from build123d import *

# Parameters (mm, degrees)
SKETCH_1_R      = 1
SKETCH_1_R_2    = 0.75
EXTRUDE_1_DEPTH = 0.5
SKETCH_1_4_R    = 0.75
SKETCH_1_4_R_2  = 0.45
EXTRUDE_2_DEPTH = 9
SKETCH_1_6_R    = 0.45
EXTRUDE_3_DEPTH = 10
CHAMFER_3_SIZE  = 0.1
CHAMFER_4_SIZE  = 0.1
CHAMFER_5_SIZE  = 0.1


with BuildPart() as part:
    # 草图1 → 凸台-拉伸1 (new body)
    with BuildSketch(Plane(origin=(0, 0, 0), x_dir=(1, 0, 0), z_dir=(0, 1, 0))):
        Circle(SKETCH_1_R)
        Circle(SKETCH_1_R_2, mode=Mode.SUBTRACT)
    extrude(amount=EXTRUDE_1_DEPTH)

    # 草图1<4> → 凸台-拉伸2 (add)
    with BuildSketch(Plane(origin=(0, 0, 0), x_dir=(1, 0, 0), z_dir=(0, 1, 0))):
        Circle(SKETCH_1_4_R)
        Circle(SKETCH_1_4_R_2, mode=Mode.SUBTRACT)
    extrude(amount=EXTRUDE_2_DEPTH)

    # 草图1<6> → 凸台-拉伸3 (add)
    with BuildSketch(Plane(origin=(0, 0, 0), x_dir=(1, 0, 0), z_dir=(0, 1, 0))):
        Circle(SKETCH_1_6_R)
    extrude(amount=EXTRUDE_3_DEPTH)

    # 倒角3
    chamfer_3_edges = [part.edges().sort_by_distance(p)[0] for p in [
        (-0.45, 10, 0),
    ]]
    chamfer(chamfer_3_edges, length=CHAMFER_3_SIZE)

    # 倒角4
    chamfer_4_edges = [part.edges().sort_by_distance(p)[0] for p in [
        (-1, 0.5, 0),
        (-0.75, 0.5, 0),
    ]]
    chamfer(chamfer_4_edges, length=CHAMFER_4_SIZE)

    # 倒角5
    chamfer_5_edges = [part.edges().sort_by_distance(p)[0] for p in [
        (-0.45, 9, 0),
        (-0.75, 9, 0),
    ]]
    chamfer(chamfer_5_edges, length=CHAMFER_5_SIZE)


solid = part.part
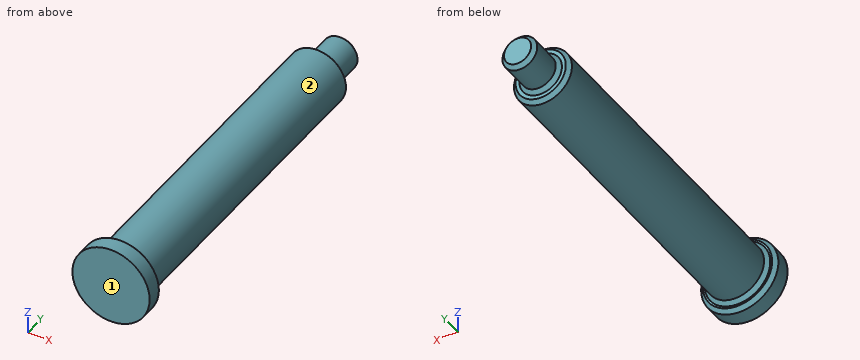
Check sheet for the modelled part. Datum: model origin and axes. Units: mm. Face numbers are marked on the shaded views. A direction names the side the tool comes from. Give positions to 0.01 mm unless a question says otherwise; leave off trailing zeros. Write each loop counter-clockwise with the first axis right and the second up, starting at its lowest first coordinate (ties: lowest second). Pieces come first, ordered by that corner, then holes. Notation, with made-up numbers: (-21, -27.75) -> (-13, -27.75) arc R24 ccw to (-13, 1.25) -> close; hole circle Ø1 at (71.5, 31). An arc over 180 degrees is marked (long way). Use one line per item in the form item = value. Start each with the question number.
1. Section check C-C (y = 9.5). Record the cut outline in (x, z), and give its area (3 significant figures).
2. Section check D-D (y = 1.25). Record the cut outline in (x, z), and give its area (3 significant figures).
3. Access from +Z, -Z, +X, -X, +Y, -Y to the whole of each face (thin tool, end or side, straight path). Record for the marked faces 1 and 2.
4. Section check A-A (z = 0). Record the cut outline in (x, y).
5. Thickness scan on line 1 along X through (y, z) = (7.75, -0.05); line 2 along Y through (x, z) = (-0.4, 0.45); line 3 along Z through (x, y) = (-0.45, 3.5). Record the ranges inside material, lowest first. Write a range as from..to.
6. Section check B-B (x = 0). Record the cut outline in (y, z), and give its area (3 significant figures).
7. Go/stop test with a flat-tipped pin: P1, Ø0.9, axis at x = -0.5, z = 0.5, coming from the +Y side. Record where the tip stops, or that it passes through.
Conclusion:
q1.outline = circle Ø0.9 at (0, 0)
q1.area = 0.636 mm²
q2.outline = circle Ø1.5 at (0, 0)
q2.area = 1.77 mm²
q3.face_1 = +Z, -Z, +X, -X, -Y
q3.face_2 = +Y
q4.outline = (-1, 0) -> (1, 0) -> (1, 0.4) -> (0.9, 0.5) -> (0.85, 0.5) -> (0.75, 0.6) -> (0.75, 8.9) -> (0.65, 9) -> (0.55, 9) -> (0.45, 9.1) -> (0.45, 9.9) -> (0.35, 10) -> (-0.35, 10) -> (-0.45, 9.9) -> (-0.45, 9.1) -> (-0.55, 9) -> (-0.65, 9) -> (-0.75, 8.9) -> (-0.75, 0.6) -> (-0.85, 0.5) -> (-0.9, 0.5) -> (-1, 0.4) -> close
q5.line_1 = -0.75..0.75
q5.line_2 = 0..9
q5.line_3 = -0.6..0.6
q6.outline = (0, -1) -> (0.4, -1) -> (0.5, -0.9) -> (0.5, -0.85) -> (0.6, -0.75) -> (8.9, -0.75) -> (9, -0.65) -> (9, -0.55) -> (9.1, -0.45) -> (9.9, -0.45) -> (10, -0.35) -> (10, 0.35) -> (9.9, 0.45) -> (9.1, 0.45) -> (9, 0.55) -> (9, 0.65) -> (8.9, 0.75) -> (0.6, 0.75) -> (0.5, 0.85) -> (0.5, 0.9) -> (0.4, 1) -> (0, 1) -> close
q6.area = 14.6 mm²
q7.P1 = 10
